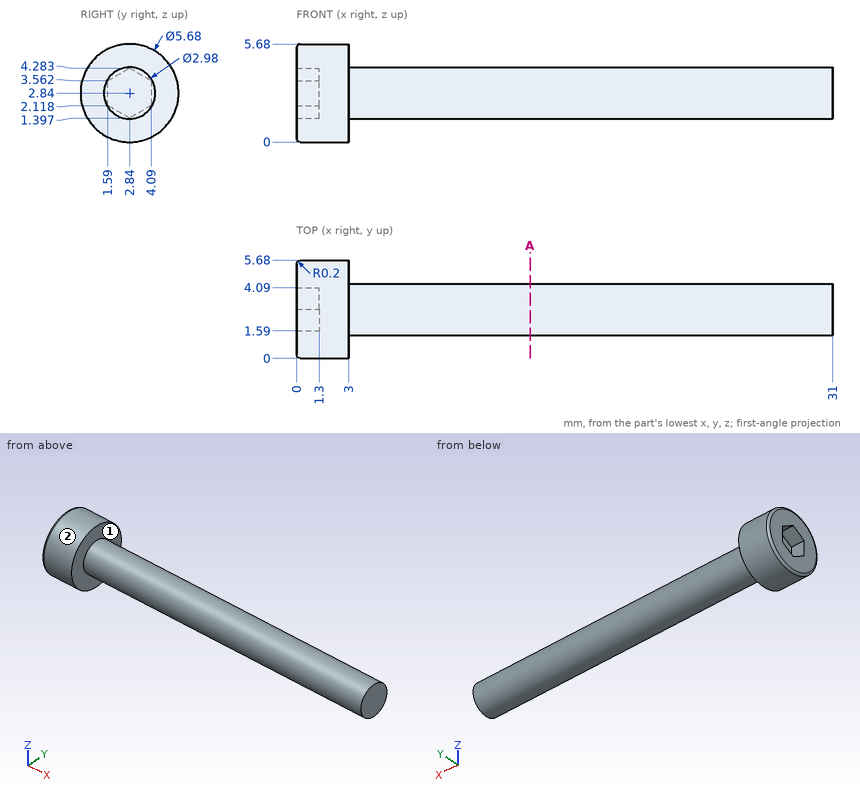
Geometry: see drawing. Coordinates: mm, zero at the bounding-box minimum. A direction names the side the tool comes from. Give positions to 0.01 mm unless a question says otherwise; leave off trailing zeros. Write each loop counter-clockwise with the first axis right and the second up, starting at its lowest first coordinate (ties: lowest second). Pieces come first, ordered by that corner, then holes. Notation, with made-up numbers: M -2.75,-21.75 L 55.25,-21.75 A25 ccw 55.25,11.25 Z; hole C 6,-2.5 d1. An arc over 180 degrees is marked long. Answer in a Markdown table with one row per item. Add a question column.
(1) Reachability of the marked faces 1 and 2 from +Z, -Z, +X, -X, +Y, -Y: full face, straight path, thin tool, end or side. Return the list, or none.
(2) First-contact query: pin 1 (0.7 mm diameter, centred on y = 3, z = 3, fed in from -X); pin 2 (1.5 mm diameter, centred on y = 5, z = 4.5, fed in from +X); pin 3 (2 mm diameter, centred on x = 18, y = 3, fed in from +Z). Flat tips, straight axial feed; report the tip coordinate or a pass-through.
(3) Ray query, line 1 (X direction, y = 2.25, z = 3.4); line 2 (X direction, y = 0.6, z = 3.8); line 3 (Z direction, x = 6, y = 2.9). Return the intervals inside material, ascending.
(4) Section A-A on x = 13.5. Return loops of the section in (y, z).
Result set:
| question | item | result |
|---|---|---|
| 1 | face 1 | +X |
| 1 | face 2 | +X, -X |
| 2 | pin 1 | stops at x = 1.3 |
| 2 | pin 2 | stops at x = 3 |
| 2 | pin 3 | stops at z = 4.33 |
| 3 | line 1 | x = 1.3 to 31 |
| 3 | line 2 | x = 0 to 3 |
| 3 | line 3 | z = 1.35 to 4.33 |
| 4 | outline | C 2.84,2.84 d2.98 |
